Part print with two shaded views. Sizes in mm from the minimum x, y, z corner. A direction names the side the tool comes from. Coordinates: 2 decimals unless noted, no trailing zeros. Order: outer loops, then holes, each group sorted by start corner. A loop starts at its lowest first (then second) coordinate and runs counter-clockwise, first axis right, second up. Notation, with made-up numbers: (-14, 81) - (8, 81) arc R13 ccw to (8, 91) - close; hole circle Ø2 at (75, 20.5). An arc over 180 degrees is marked (long way). One line per item, written item: value.
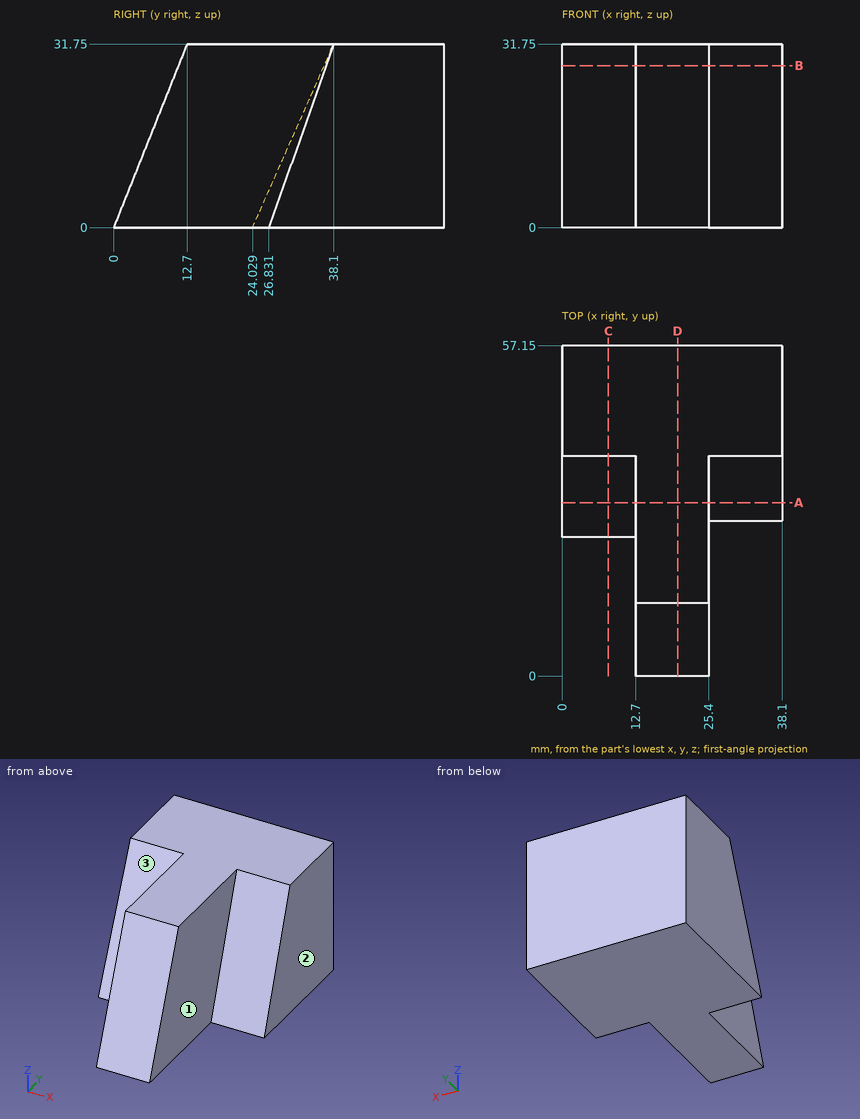
1. Band-saw the part on A-A, the plane y = 30. Give the cut face in (x, z), and give its area (3 significant figures).
Values found:
outline: (0, 0) - (38.1, 0) - (38.1, 8.93) - (25.4, 8.93) - (25.4, 31.75) - (12.7, 31.75) - (12.7, 13.47) - (0, 13.47) - close
area: 688 mm2
2. Band-saw the part on D-D, the plane x = 20. Give the cut face in (y, z), and give its area (3 significant figures).
Values found:
outline: (0, 0) - (57.15, 0) - (57.15, 31.75) - (12.7, 31.75) - close
area: 1,610 mm2
3. 3-axis set-ups, long thin cutter, end or side, ignore diameter. For the marked faces 1, 2 and 3: which of +Z, -Z, +X, -X, +Y, -Y reach the whole face in a straight line?
Values found:
face 1: +Z, +X, -Y
face 2: +Z, -Z, +X, +Y, -Y
face 3: +Z, -X, -Y
4. Band-saw the part on B-B, the plane z = 28. Give the cut face in (x, y).
Values found:
outline: (0, 36.44) - (12.7, 36.44) - (12.7, 11.2) - (25.4, 11.2) - (25.4, 36.77) - (38.1, 36.77) - (38.1, 57.15) - (0, 57.15) - close
5. Band-saw the part on C-C, the plane x = 8. Give the cut face in (y, z).
Values found:
outline: (24.03, 0) - (57.15, 0) - (57.15, 31.75) - (38.1, 31.75) - close
6. Probe line 1 along X through (y, z) = (14, 29.5); line 2 along Y through (x, z) = (29.5, 8.5); line 3 along Z through (x, y) = (9.5, 31). List the from-to ranges inside material, lowest first.
Values found:
line 1: x = 12.7 to 25.4
line 2: y = 29.85 to 57.15
line 3: z = 0 to 15.73
7. Flat gauge pins, fed straight in: P1, Ø2, axis at y = 17, z = 28, coming from the +X side; P2, Ø10, axis at y = 20.5, z = 14, coming from the -X side; P3, Ø12, axis at x = 23, z = 23.5, coming from the -Y side. Where does each tip first touch, or does it go through?
Values found:
P1: stops at x = 25.4
P2: stops at x = 12.7
P3: stops at y = 7
